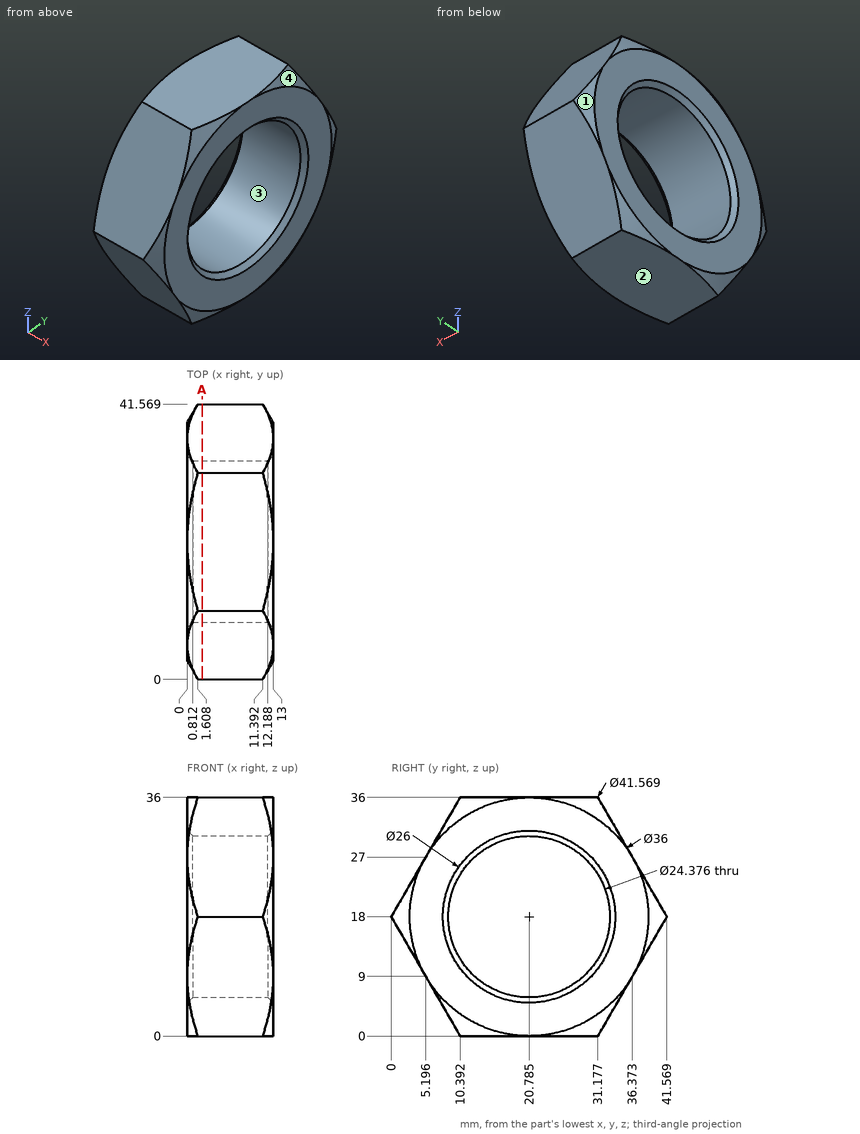
Job drawing, mm, ordinate dimensions from the low corner. One solid piece. Coordinates: 2 decimals unless noted, no trailing zeros. Order: outer loops, then holes, each group sorted by start corner. A loop starts at its lowest first (then second) coordinate and runs counter-clockwise, first axis right, second up. Notation, with made-up numbers: (-10.75, 75.25) - (34.25, 75.25) arc R27 cw to (34.25, 114.25) - close; hole circle Ø8 at (-23, 77). An arc over 180 degrees is marked (long way). Return JSON: item names as keys, results as strings. Group by question number.
1) Mould opens along Z. For the marked faces 1, 2, 3 and 4 say: released by +Z, released by -Z, zero draft, split by the parting line, or undercut.
2) Flat gauge pins, fed straight in: P1, Ø1.5, axis at x = 4, z = 8.5, coming from the +Y side; P2, Ø6, axis at x = 6, z = 30.5, coming from the -Y side (1 decimal); P3, Ø10, axis at y = 10.5, z = 21.5, coming from the -X side; P4, Ø1, axis at x = 6.5, z = 4.5, coming from the +Y side. Where does each tip first touch, or does it go through?
3) Probe line 1 (Z direction, x = 10, y = 21); line 2 (Y direction, x = 11, z = 14); line 3 (Z direction, x = 3.5, y = 29.5). List the from-to ranges inside material, lowest first. Write a range as from..to.
4) Saw through at A-A, the plane x = 2.25. Write the cut outline in (y, z) (1 decimal), plus the area to 3 significant figures.
Values found:
{
 "1": {"face 1": "split by the parting line", "face 2": "released by -Z", "face 3": "undercut", "face 4": "released by +Z"},
 "2": {"P1": "stops at y = 36.52", "P2": "stops at y = 5.5", "P3": "stops at x = 0", "P4": "stops at y = 34.06"},
 "3": {"line 1": "z = 0..5.81, 30.19..36", "line 2": "y = 2.31..9.27, 32.3..39.26", "line 3": "z = 0..9.48, 26.52..36"},
 "4": {"outline": "(0, 18) - (10.4, 0) - (31.2, 0) - (41.6, 18) - (31.2, 36) - (10.4, 36) - close; hole circle Ø24.4 at (20.8, 18)", "area": "656 mm²"}
}
